from build123d import *

# Parameters (mm, degrees)
SKETCH1_W           = 82
SKETCH1_H           = 56.6
SKETCH1_R           = 3.5
SKETCH1_R_2         = 1.5
BOSS_EXTRUDE1_DEPTH = 1.5
SKETCH1_3_R         = 3.5
SKETCH1_3_R_2       = 1.5
BOSS_EXTRUDE2_DEPTH = 5.5
FILLET1_R           = 2
FILLET2_R           = 4


with BuildPart() as part:
    # Sketch1 → Boss-Extrude1 (new body)
    # profile 1 of 11: a face of its own
    with BuildSketch(Plane(origin=(0, 0, 0), x_dir=(1, 0, 0), z_dir=(0, 1, 0))):
        Rectangle(SKETCH1_W, SKETCH1_H)
        with Locations((-35, -22.3)):
            Circle(SKETCH1_R, mode=Mode.SUBTRACT)
        with Locations((35, -22.3)):
            Circle(SKETCH1_R, mode=Mode.SUBTRACT)
        with Locations((35, 22.3)):
            Circle(SKETCH1_R, mode=Mode.SUBTRACT)
        with Locations((-35, 22.3)):
            Circle(SKETCH1_R, mode=Mode.SUBTRACT)
    # profile 2 of 11: a face of its own
    with BuildSketch(Plane(origin=(0, 0, 0), x_dir=(1, 0, 0), z_dir=(0, 1, 0))):
        with BuildLine():
            ThreePointArc((-46.333333333, -5.185449729), (-42.468027353, -8.109119908), (-41, -12.727922061))
            Line((-41, -12.727922061), (-41, 12.727922061))
            ThreePointArc((-41, 12.727922061), (-42.468027353, 8.109119908), (-46.333333333, 5.185449729))
            ThreePointArc((-46.333333333, 5.185449729), (-50, 0), (-46.333333333, -5.185449729))
        make_face()
        with Locations(Location((-44.5, 0, 0), (0, 0, 270))):
            Circle(SKETCH1_R_2, mode=Mode.SUBTRACT)
    # profile 3 of 11: a face of its own
    with BuildSketch(Plane(origin=(0, 0, 0), x_dir=(1, 0, 0), z_dir=(0, 1, 0))):
        with BuildLine():
            Line((41, 12.727922061), (41, -12.727922061))
            ThreePointArc((41, -12.727922061), (42.468027353, -8.109119908), (46.333333333, -5.185449729))
            ThreePointArc((46.333333333, -5.185449729), (50, 0), (46.333333333, 5.185449729))
            ThreePointArc((46.333333333, 5.185449729), (42.468027353, 8.109119908), (41, 12.727922061))
        make_face()
        with Locations(Location((44.5, 0, 0), (0, 0, 270))):
            Circle(SKETCH1_R_2, mode=Mode.SUBTRACT)
    # profile 4 of 11: a face of its own
    with BuildSketch(Plane(origin=(0, 0, 0), x_dir=(1, 0, 0), z_dir=(0, 1, 0))):
        with Locations((-35, -22.3)):
            Circle(SKETCH1_R)
        with Locations((-35, -22.3)):
            Circle(SKETCH1_R_2, mode=Mode.SUBTRACT)
    # profile 5 of 11: a face of its own
    with BuildSketch(Plane(origin=(0, 0, 0), x_dir=(1, 0, 0), z_dir=(0, 1, 0))):
        with Locations((-35, -22.3)):
            Circle(SKETCH1_R_2)
    # profile 6 of 11: a face of its own
    with BuildSketch(Plane(origin=(0, 0, 0), x_dir=(1, 0, 0), z_dir=(0, 1, 0))):
        with Locations((35, -22.3)):
            Circle(SKETCH1_R)
        with Locations((35, -22.3)):
            Circle(SKETCH1_R_2, mode=Mode.SUBTRACT)
    # profile 7 of 11: a face of its own
    with BuildSketch(Plane(origin=(0, 0, 0), x_dir=(1, 0, 0), z_dir=(0, 1, 0))):
        with Locations((35, -22.3)):
            Circle(SKETCH1_R_2)
    # profile 8 of 11: a face of its own
    with BuildSketch(Plane(origin=(0, 0, 0), x_dir=(1, 0, 0), z_dir=(0, 1, 0))):
        with Locations((35, 22.3)):
            Circle(SKETCH1_R)
        with Locations((35, 22.3)):
            Circle(SKETCH1_R_2, mode=Mode.SUBTRACT)
    # profile 9 of 11: a face of its own
    with BuildSketch(Plane(origin=(0, 0, 0), x_dir=(1, 0, 0), z_dir=(0, 1, 0))):
        with Locations((35, 22.3)):
            Circle(SKETCH1_R_2)
    # profile 10 of 11: a face of its own
    with BuildSketch(Plane(origin=(0, 0, 0), x_dir=(1, 0, 0), z_dir=(0, 1, 0))):
        with Locations((-35, 22.3)):
            Circle(SKETCH1_R)
        with Locations((-35, 22.3)):
            Circle(SKETCH1_R_2, mode=Mode.SUBTRACT)
    # profile 11 of 11: a face of its own
    with BuildSketch(Plane(origin=(0, 0, 0), x_dir=(1, 0, 0), z_dir=(0, 1, 0))):
        with Locations((-35, 22.3)):
            Circle(SKETCH1_R_2)
    extrude(amount=BOSS_EXTRUDE1_DEPTH)

    # Sketch1<3> → Boss-Extrude2 (add)
    # profile 1 of 4: a face of its own
    with BuildSketch(Plane(origin=(0, 0, 0), x_dir=(1, 0, 0), z_dir=(0, 1, 0))):
        with Locations(Location((-35, 22.3, 0), (0, 0, 270))):
            Circle(SKETCH1_3_R)
        with Locations(Location((-35, 22.3, 0), (0, 0, 270))):
            Circle(SKETCH1_3_R_2, mode=Mode.SUBTRACT)
    # profile 2 of 4: a face of its own
    with BuildSketch(Plane(origin=(0, 0, 0), x_dir=(1, 0, 0), z_dir=(0, 1, 0))):
        with Locations(Location((35, 22.3, 0), (0, 0, 270))):
            Circle(SKETCH1_3_R)
        with Locations(Location((35, 22.3, 0), (0, 0, 270))):
            Circle(SKETCH1_3_R_2, mode=Mode.SUBTRACT)
    # profile 3 of 4: a face of its own
    with BuildSketch(Plane(origin=(0, 0, 0), x_dir=(1, 0, 0), z_dir=(0, 1, 0))):
        with Locations(Location((35, -22.3, 0), (0, 0, 270))):
            Circle(SKETCH1_3_R)
        with Locations(Location((35, -22.3, 0), (0, 0, 270))):
            Circle(SKETCH1_3_R_2, mode=Mode.SUBTRACT)
    # profile 4 of 4: a face of its own
    with BuildSketch(Plane(origin=(0, 0, 0), x_dir=(1, 0, 0), z_dir=(0, 1, 0))):
        with Locations(Location((-35, -22.3, 0), (0, 0, 270))):
            Circle(SKETCH1_3_R)
        with Locations(Location((-35, -22.3, 0), (0, 0, 270))):
            Circle(SKETCH1_3_R_2, mode=Mode.SUBTRACT)
    extrude(amount=BOSS_EXTRUDE2_DEPTH)

    # Fillet1
    fillet1_edges = [part.edges().sort_by_distance(p)[0] for p in [
        (-35, 1.5, -25.8),
        (35, 1.5, -25.8),
        (35, 1.5, 18.8),
        (-35, 1.5, 18.8),
    ]]
    fillet(fillet1_edges, radius=FILLET1_R)

    # Fillet2
    fillet2_edges = [part.edges().sort_by_distance(p)[0] for p in [
        (-41, 0.75, 28.3),
        (-41, 0.75, -28.3),
        (41, 0.75, -28.3),
        (41, 0.75, 28.3),
    ]]
    fillet(fillet2_edges, radius=FILLET2_R)


solid = part.part
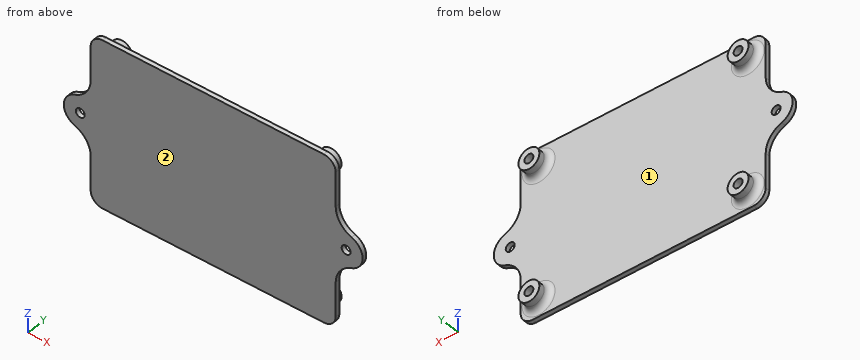
Verification items for the finished model (mm, model axes). Face numbers are marked on the shaded views. Round coordinates to 2 decimals unless told otherwise and drop trailing zeros. Loops run counter-clockwise (first coordinate to the right, second up) from the corner with the lowest first, then second, coordinate; pieces in that order, holes last. Notation, with made-up numbers: (42.25, 47) - (72.25, 47) arc R19 cw to (72.25, 72) - close; hole circle Ø1 at (28.5, 13.5). An arc over 180 degrees is marked (long way). Answer in a Markdown table with one row per item. Add a question column.
Q1. Section check B-B on z = 0. Enter the section's corners in (x, y).
Q2. Section check D-D on x = -28.5. Enter the section's corners in (y, z).
Q3. Material ranges on line 1 (X direction, y = 0.8, z = 0); line 2 (X direction, y = 3.25, z = 22.3); line 3 (Z direction, x = -35, y = 2.65), recorded low to high.
Q4. Release check for a two-part mould opening along X. For the marked faces 1 and 2 record: pulls with the +X half, pulls with the -X half, needs draft (parallel to the pull), parting line crosses it, or undercut.
Q5. Gauge pin test, flat ends, axial feed: pin 1 (0.8 mm diameter, centred on y = 0.5, z = 16.5, fed in from +X); pin 2 (1.5 mm diameter, centred on x = -34.5, z = 22.5, fed in from +Y); pin 3 (1.2 mm diameter, centred on y = 1, z = -21.5, fed in from -X). Record the tip position at first contact, or that the pin passes through.
Q6. Section check C-C on z = -22.3. Enter the section's corners in (x, y), plus the area to 3 significant figures.
Q7. Section check A-A on x = 44.5. Enter the section's corners in (y, z), plus the area to 3 significant figures.
Found:
| question | item | result |
|---|---|---|
| 1 | outline | (-50, 0) - (-46, 0) - (-46, 1.5) - (-50, 1.5) - close; (-43, 0) - (43, 0) - (43, 1.5) - (-43, 1.5) - close; (46, 0) - (50, 0) - (50, 1.5) - (46, 1.5) - close |
| 2 | outline | (0, -28.3) - (1.5, -28.3) - (1.5, 28.3) - (0, 28.3) - close |
| 3 | line 1 | x = -50 to -46, -43 to 43, 46 to 50 |
| 3 | line 2 | x = -38.52 to -36.5, -33.5 to -31.48, 31.48 to 33.5, 36.5 to 38.52 |
| 3 | line 3 | z = -25.99 to -23.8, -20.8 to -18.61, 18.61 to 20.8, 23.8 to 25.99 |
| 4 | face 1 | undercut |
| 4 | face 2 | needs draft |
| 5 | pin 1 | stops at x = 41 |
| 5 | pin 2 | stops at y = 1.5 |
| 5 | pin 3 | stops at x = -41 |
| 6 | outline | (-41, 0) - (41, 0) - (41, 1.5) - (40.5, 1.5) arc R2 cw to (38.5, 3.5) - (38.5, 5.5) - (36.5, 5.5) - (36.5, 1.5) - (33.5, 1.5) - (33.5, 5.5) - (31.5, 5.5) - (31.5, 3.5) arc R2 cw to (29.5, 1.5) - (-29.5, 1.5) arc R2 cw to (-31.5, 3.5) - (-31.5, 5.5) - (-33.5, 5.5) - (-33.5, 1.5) - (-36.5, 1.5) - (-36.5, 5.5) - (-38.5, 5.5) - (-38.5, 3.5) arc R2 cw to (-40.5, 1.5) - (-41, 1.5) - close |
| 6 | area | 158 mm² |
| 7 | outline | (0, -6.11) - (1.5, -6.11) - (1.5, -1.5) - (0, -1.5) - close; (0, 1.5) - (1.5, 1.5) - (1.5, 6.11) - (0, 6.11) - close |
| 7 | area | 13.8 mm² |
